from build123d import *

# Parameters (mm, degrees)
SKETCH1_W           = 45
SKETCH1_H           = 45
BOSS_EXTRUDE1_DEPTH = 320
CUT_EXTRUDE3_DEPTH  = 50
SKETCH3_W           = 45
SKETCH3_H           = 45
CUT_EXTRUDE4_DEPTH  = 20


with BuildPart() as part:
    # Sketch1 → Boss-Extrude1 (new body)
    with BuildSketch(Plane.XY):
        Rectangle(SKETCH1_W, SKETCH1_H)
    extrude(amount=BOSS_EXTRUDE1_DEPTH)

    # Sketch2 → Cut-Extrude3 (cut)
    with BuildSketch(Plane.ZY.offset(22.5)):
        Polygon((290, 17.5), (290, -17.5), (305, -17.5), (320, -2.5), (320, 2.5), (305, 17.5), align=None)
        Polygon((320, 22.5), (307.928932188, 22.5), (320, 10.428932188), align=None)
        Polygon((320, -10.428932188), (307.928932188, -22.5), (320, -22.5), align=None)
    extrude(amount=-CUT_EXTRUDE3_DEPTH, mode=Mode.SUBTRACT)

    # Sketch3 → Cut-Extrude4 (cut)
    with BuildSketch(Plane(origin=(0, 0, 0), x_dir=(-1, 0, 0), z_dir=(0, 0, -1))):
        Rectangle(SKETCH3_W, SKETCH3_H)
    extrude(amount=-CUT_EXTRUDE4_DEPTH, mode=Mode.SUBTRACT)


solid = part.part
The model under review builds one solid part; all positions refer to its coordinate system, in mm. A direction names the side the tool comes from. Give positions to 0.01 mm unless a question says otherwise; leave off trailing zeros. Order: outer loops, then holes, each group sorted by start corner. A loop starts at its lowest first (then second) coordinate and runs counter-clockwise, first axis right, second up. Notation, with made-up numbers: M 35.25,24 L 80.25,24 A13 ccw 80.25,30 Z; hole C -25.5,74.5 d4. An arc over 180 degrees is marked long. Use one line per item in the form item = value. Start each with the question number.
Item 1: To check wall thickness, follow line 1 along Z through (x, y) = (-5, 11); line 2 along Z through (x, y) = (6, 12); line 3 along Z through (x, y) = (7, -19). State the ranges of each line that lie inside material, in increasing order. Write a range as from..to.
Item 2: Insertion check: pin 1 Ø6 at (x, y) = (8, 11) entering from +Z. The pin has a flat end and moves straight along its axis. Give the tip position at first contact, or say it passes through.
Item 3: The part is to be moulded in two halves that separate along Z. For faces 3 (the flat face through (0, 0, 20)), 4 (the flat face through (0, -22.5, 162)), 5 (the flat face through (-0.3, -10.1, 312.4)), say which applies: pulls with the +Z half, pulls with the -Z half, needs draft (parallel to the pull), parting line crosses it, or undercut.
Item 4: For faces 1 (the flat face through (0, -6, 320)), 2 (the flat face through (0, -17.5, 297)), list the 3-axis set-ups (+Z, -Z, +X, -X, +Y, -Y) from which the entire face can be reached by the end or side of a thin tool; tool diameter is ignored.
Item 5: We need section A-A on x = -14.5. Give the boundary of the cut face in (y, z).
Item 6: We need section B-B on y = 14.5. Give the boundary of the cut face in (x, z), plus the area to 3 significant figures.
Completed:
q1.line_1 = 20..290, 311.5..319.43
q1.line_2 = 20..290, 310.5..318.43
q1.line_3 = 20..311.43
q2.pin_1 = 320
q3.face_3 = pulls with the -Z half
q3.face_4 = needs draft
q3.face_5 = undercut
q4.face_1 = +Z, +X, -X, +Y, -Y
q4.face_2 = +X, -X
q5.outline = M -22.5,20 L 22.5,20 L 22.5,307.93 L 10.43,320 L 2.5,320 L 17.5,305 L 17.5,290 L -17.5,290 L -17.5,305 L -2.5,320 L -10.43,320 L -22.5,307.93 Z
q6.outline = M -22.5,20 L 22.5,20 L 22.5,290 L -22.5,290 Z; M -22.5,308 L 22.5,308 L 22.5,315.93 L -22.5,315.93 Z
q6.area = 12,500 mm²
